Autodesk Inventor part; units mm, degrees
ref_plane "Work Plane1" through (0, 5, 0) normal (0, 1, 0) x (-1, 0, 0)
ref_plane "YZ Plane" through (0, 0, 0) normal (1, 0, 0) x (0, 1, 0)
ref_plane "XY Plane" through (0, 0, 0) normal (0, 0, 1) x (1, 0, 0)
sketch "Sketch1" plane through (0, 0, 0) normal (0, 0, 1) x (1, 0, 0)
  line L0 (0, 0) -> (43, 0)
  arc A0 (43, 0) -> (40.5, 2.5) centre (40.5, 0) ccw
  line L1 (40.5, 2.5) -> (35, 2.5)
  line L2 (35, 2.5) -> (35, 1.25)
  line L3 (35, 1.25) -> (0, 1.25)
  line L4 (0, 1.25) -> (0, 0)
  point P0 (0, 0.625)
  dimension "d0" = 2.5
  dimension "d1" = 5.5
  dimension "d2" = 2.5
  dimension "d3" = 40.5
revolve "Revolution1" add sketch "Sketch1" angle 360 about axis through (0, 0, 0) along (1, 0, 0)
ref_plane "Work Plane1" through (0, 5, 0) normal (0, 1, 0) x (-1, 0, 0)
sketch "Sketch2" plane through (0, 5, 0) normal (0, 1, 0) x (-1, 0, 0)
  arc A0 (-40.5, 2.5) -> (-40.5, -2.5) centre (-40.5, 0) ccw
  line L0 (-35, -1.25) -> (-35, 1.25) construction
  line L1 (-40.5, 2.5) -> (-40.5, -2.5) construction
  line L2 (-35, 2.5) -> (-35, -2.5)
  line L3 (-35, -1.25) -> (-42.6651, -1.25)
  line L4 (-35, 1.25) -> (-42.6651, 1.25)
  line L5 (-35, -2.5) -> (-40.5, -2.5)
  line L6 (-35, 2.5) -> (-40.5, 2.5)
  point P0 (0, 0)
  point P1 (-35, 0)
  dimension "d6" = 2.5
  dimension "d9" = 2.5
  dimension "d10" = 1.25
extrude "Extrusion2" cut sketch "Sketch2" against normal blind 10 contours L6 L2 L4 A0 | L3 L2 L5 A0
sketch "Sketch3" plane through (40.5, -2.1651, -1.25) normal (0, 0, -1) x (-1, 0, 0)
  arc A0 (0, 4.3301) -> (0, 0) centre (0, 2.1651) ccw
  point P0 (40.5, 2.1651)
hole "Hole1" at (40.5, 0, -1.25) direction (0, 0, 1) diameter 2.6 depth 2.5
properties part number "21.2"
Work out the finished part from the listing and answer in its coordinate system (mm). A direction names the side the tool comes from. Give positions to 0.01 mm unless a question says otherwise; leave off trailing zeros. Order: outer loops, then holes, each group sorted by start corner. A loop starts at its lowest first (then second) coordinate and runs counter-clockwise, first axis right, second up. Notation, with made-up numbers: (45, -15.5) -> (102, -15.5) arc R28 cw to (102, 5.5) -> close; hole circle Ø7 at (-33.75, 5). An arc over 180 degrees is marked (long way). Answer as CSV lines item,"result". Start each with the question number.
(1) Consider line 1 along X through (y, z) = (0, -0.05); line 2 along Y through (x, z) = (40.5, 0.1); line 3 along X through (y, z) = (-0.5, -0.4). Determine where each line is inside the solid, lowest interval first.
(2) Section C-C, the plane x = 9 is taken. Write down the section's boundary in (y, z).
(3) Each of these flat-tipped pins is pushed along its axis until it touches: pin 1 Ø1.2 at (y, z) = (-1.5, 0.5) entering from -X; pin 2 Ø1.5 at (y, z) = (1, 1) entering from +X; pin 3 Ø1 at (x, z) = (32.5, -0.5) entering from +Y. Where does it stop, or does it pass through?
(4) Section B-B, the plane x = 36.5 is taken. Write down the section's boundary in (y, z).
(5) Which of the six approach directions +Z, -Z, +X, -X, +Y, -Y give full straight-line access (tool end or side, diameter ignored) to faces 1 (the flat face through (35, 2, 0)), 2 (the flat face through (0, 0, 0))?
(6) Section A-A, the plane z = -0.75 is taken. Write down the section's boundary in (x, y).
(7) For a pull along Y with two mould halves and no side action, classify faces 3 (the cylindrical face through (37.7, 2.5, 0)), 4 (the cylindrical face through (17.26, -0.27, 1.22)), 5 (the cylindrical face through (39.21, -0.17, 0.02)), 6 (the flat face through (38, 0, -1.25)) as released by +Y, released by -Y, zero draft, split by the parting line, or undercut.
Entries:
1,line 1,"0 to 39.2, 41.8 to 43"
1,line 2,"-2.5 to -1.3, 1.3 to 2.5"
1,line 3,"0 to 39.3, 41.7 to 42.92"
2,outline,"circle Ø2.5 at (0, 0)"
3,pin 1,"x = 0"
3,pin 2,"x = 42.91"
3,pin 3,"y = 1.25"
4,outline,"(-2.17, -1.25) -> (2.17, -1.25) arc R2.5 ccw to (2.17, 1.25) -> (-2.17, 1.25) arc R2.5 ccw to start"
5,face 1,"-X, +Y"
5,face 2,"+Z, -Z, -X, +Y, -Y"
6,outline,"(0, -1) -> (35, -1) -> (35, -2.38) -> (40.5, -2.38) arc R2.38 ccw to (40.5, 2.38) -> (35, 2.38) -> (35, 1) -> (0, 1) -> close; hole circle Ø2.6 at (40.5, 0)"
7,face 3,"released by +Y"
7,face 4,"split by the parting line"
7,face 5,"undercut"
7,face 6,"zero draft"
